from build123d import *

# Parameters (mm, degrees)
F1_DEPTH = 40.64
F3_DEPTH = 38.608
F5_DEPTH = 4.7752
F6_R     = 1.35255
F7_DEPTH = 4.7752


# Not quite as in the source:
# - a feature names something its author has since deleted; it is built from what else it names


with BuildPart() as f1:
    # F0 (on Top) → F1 (new body)
    with BuildSketch(Plane.XY):
        with BuildLine():
            ThreePointArc((0, 2), (0.5857864376, 0.5857864376), (2, 0))
            Line((2, 0), (75.216, 0))
            ThreePointArc((75.216, 0), (76.6302135624, 0.5857864376), (77.216, 2))
            Line((77.216, 2), (77.216, 49.816))
            ThreePointArc((77.216, 49.816), (76.6302135624, 51.2302135624), (75.216, 51.816))
            Line((75.216, 51.816), (2, 51.816))
            ThreePointArc((2, 51.816), (0.5857864376, 51.2302135624), (0, 49.816))
            Line((0, 49.816), (0, 2))
        make_face()
    extrude(amount=F1_DEPTH)

    # F2 (on face) → F3 (cut)
    with BuildSketch(Plane.XY.offset(40.64)):
        with BuildLine():
            Line((74.416, 50.016), (2.8, 50.016))
            ThreePointArc((2.8, 50.016), (2.0928932188, 49.7231067812), (1.8, 49.016))
            Line((1.8, 49.016), (1.8, 2.8))
            ThreePointArc((1.8, 2.8), (2.0928932188, 2.0928932188), (2.8, 1.8))
            Line((2.8, 1.8), (74.416, 1.8))
            ThreePointArc((74.416, 1.8), (75.1231067812, 2.0928932188), (75.416, 2.8))
            Line((75.416, 2.8), (75.416, 49.016))
            ThreePointArc((75.416, 49.016), (75.1231067812, 49.7231067812), (74.416, 50.016))
        make_face()
    extrude(amount=-F3_DEPTH, mode=Mode.SUBTRACT)

    # F4 (on face) → F5 (join)
    with BuildSketch(Plane(origin=(0, 0, 0), x_dir=(1, 0, 0), z_dir=(0, 0, -1))):
        with BuildLine():
            ThreePointArc((77.216, -2), (76.6302135624, -0.5857864376), (75.216, 0))
            Line((75.216, 0), (71.406, 0))
            Line((71.406, 0), (71.406, -2))
            ThreePointArc((71.406, -2), (72.5219231637, -4.6940768363), (75.216, -5.81))
            Line((75.216, -5.81), (77.216, -5.81))
            Line((77.216, -5.81), (77.216, -2))
        make_face()
        with BuildLine():
            Line((71.406, -49.816), (71.406, -51.816))
            Line((71.406, -51.816), (75.216, -51.816))
            ThreePointArc((75.216, -51.816), (76.6302135624, -51.2302135624), (77.216, -49.816))
            Line((77.216, -49.816), (77.216, -46.006))
            Line((77.216, -46.006), (75.216, -46.006))
            ThreePointArc((75.216, -46.006), (72.5219231637, -47.1219231637), (71.406, -49.816))
        make_face()
        with BuildLine():
            ThreePointArc((5.81, -49.816), (4.6940768363, -47.1219231637), (2, -46.006))
            Line((2, -46.006), (0, -46.006))
            Line((0, -46.006), (0, -49.816))
            ThreePointArc((0, -49.816), (0.5857864376, -51.2302135624), (2, -51.816))
            Line((2, -51.816), (5.81, -51.816))
            Line((5.81, -51.816), (5.81, -49.816))
        make_face()
        with BuildLine():
            Line((5.81, 0), (2, 0))
            ThreePointArc((2, 0), (0.5857864376, -0.5857864376), (0, -2))
            Line((0, -2), (0, -5.81))
            Line((0, -5.81), (2, -5.81))
            ThreePointArc((2, -5.81), (4.6940768363, -4.6940768363), (5.81, -2))
            Line((5.81, -2), (5.81, 0))
        make_face()
    extrude(amount=-F5_DEPTH)

    # F6 (on face) → F7 (cut, through all)
    with BuildSketch(Plane(origin=(0, 0, 0), x_dir=(1, 0, 0), z_dir=(0, 0, -1))):
        with Locations((73.8658709242, -3.3501290758)):
            Circle(F6_R)
        with Locations((3.3501290758, -3.3501290758)):
            Circle(F6_R)
        with Locations((3.3501290758, -48.4658709242)):
            Circle(F6_R)
        with Locations((73.8658709242, -48.4658709242)):
            Circle(F6_R)
    extrude(amount=-F7_DEPTH, mode=Mode.SUBTRACT)


solid = f1.part
CAD build for the part. Positions are in the model's coordinates, mm. A direction names the side the tool comes from. Coordinates: 2 decimals unless noted, no trailing zeros. Write each loop counter-clockwise with the first axis right and the second up, starting at its lowest first coordinate (ties: lowest second). Pieces come first, ordered by that corner, then holes. Notation, with made-up numbers: (12.5, 79.5) - (61.5, 79.5) arc R17 ccw to (61.5, 92.5) - close; hole circle Ø10 at (24, 27). An arc over 180 degrees is marked (long way). Use a Markdown table: item, result. Add a question column.
Item 1: Band-saw the part on B-B, the plane y = 17. Give the cut face in (x, z), and give its area (3 significant figures).
Item 2: Band-saw the part on A-A, the plane z = 7. Give the cut face in (x, y).
Item 3: 3-axis set-ups, long thin cutter, end or side, ignore diameter. For faces 5 (the face through (72.49, 4.66, 3.38)), 6 (the face through (0.57, 0.6, 20.04)): which of +Z, -Z, +X, -X, +Y, -Y reach the whole face in a straight line?
Item 4: Flat gauge pins, fed straight in: pin 1 (2 mm diameter, centred on x = 73.87, y = 3.35, fed in from -Z); pin 2 (4.5 mm diameter, centred on x = 3, y = 49, fed in from +Z); pin 3 (6 mm diameter, centred on x = 37, y = 25.5, fed in from +Z); pin 4 (2 mm diameter, centred on x = 74, y = 4.5, fed in from +Z). Where does each tip first touch, or does it go through?
Item 5: Drill centre lines: L1, parallel to X at y = 19.5, z = 12.5; L2, parallel to Y at x = 30.5, z = 11.5; L3, parallel to Z at x = 52, y = 12. Where is each one in solid material? Low to high. Write a range as from..to.
Item 6: Band-saw the part on C-C, the plane x = 39. Give the cut face in (y, z).
Item 7: Mould opens along Y. For faces 1 (the face through (38, 1.8, 22)), 2 (the face through (0.601, 51.246, 20.036)), 3 (the face through (38, 26, 0)), 4 (the face through (39, 50.016, 22)) say: pulls with the +Y half, pulls with the -Y half, needs draft (parallel to the pull), parting line crosses it, or undercut.
Numbers:
| question | item | result |
|---|---|---|
| 1 | outline | (0, 0) - (77.22, 0) - (77.22, 40.64) - (75.42, 40.64) - (75.42, 2.03) - (1.8, 2.03) - (1.8, 40.64) - (0, 40.64) - close |
| 1 | area | 296 mm2 |
| 2 | outline | (0, 2) arc R2 ccw to (2, 0) - (75.22, 0) arc R2 ccw to (77.22, 2) - (77.22, 49.82) arc R2 ccw to (75.22, 51.82) - (2, 51.82) arc R2 ccw to (0, 49.82) - close; hole (1.8, 2.8) arc R1 ccw to (2.8, 1.8) - (74.42, 1.8) arc R1 ccw to (75.42, 2.8) - (75.42, 49.02) arc R1 ccw to (74.42, 50.02) - (2.8, 50.02) arc R1 ccw to (1.8, 49.02) - close |
| 3 | face 5 | +Z |
| 3 | face 6 | +Z, -Z, -X, -Y |
| 4 | pin 1 | through |
| 4 | pin 2 | z = 40.64 |
| 4 | pin 3 | z = 2.03 |
| 4 | pin 4 | z = 4.78 |
| 5 | L1 | 0..1.8, 75.42..77.22 |
| 5 | L2 | 0..1.8, 50.02..51.82 |
| 5 | L3 | 0..2.03 |
| 6 | outline | (0, 0) - (51.82, 0) - (51.82, 40.64) - (50.02, 40.64) - (50.02, 2.03) - (1.8, 2.03) - (1.8, 40.64) - (0, 40.64) - close |
| 7 | face 1 | undercut |
| 7 | face 2 | pulls with the +Y half |
| 7 | face 3 | needs draft |
| 7 | face 4 | undercut |
